from build123d import *

# Parameters (mm, degrees)
ESKIZ_KONTUR_W        = 3.2
ESKIZ_KONTUR_H        = 8.2
PLASTINA_DEPTH        = 3
OTVERSTIYA_DEPTH      = 49.541218109
OTVERSTIYA_DEPTH_BACK = 49.541218109
ESKIZ_OTVERSTIYA_R    = 0.75
ESKIZ_OTVERSTIYA_R_2  = 4.5
ESKIZ_OTVERSTIYA_R_3  = 3
ESKIZ_OTVERSTIYA_R_4  = 1.65


with BuildPart() as part:
    # Eskiz_kontur → Plastina (new body)
    with BuildSketch(Plane.XY):
        with BuildLine():
            Line((41.499998426, -24.999999723), (25.999998426, -24.999999723))
            Line((25.999998426, -24.999999723), (-4.976321574, -10.919529723))
            ThreePointArc((-4.976321574, -10.919529723), (-11.817691954, 2.083782335), (-0.94151, 11.96301))
            Line((-0.94151, 11.96301), (26, 14))
            Line((26, 14), (41.499998426, 14))
            Line((41.499998426, 14), (41.499998426, -24.999999723))
        make_face()
        with Locations((36.5, -16)):
            Rectangle(ESKIZ_KONTUR_W, ESKIZ_KONTUR_H, mode=Mode.SUBTRACT)
        with Locations((36.5, 6)):
            Rectangle(ESKIZ_KONTUR_W, ESKIZ_KONTUR_H, mode=Mode.SUBTRACT)
    extrude(amount=PLASTINA_DEPTH)

    # Eskiz_otverstiya → Otverstiya (cut, two sides: drawn at the far end of the back side and taken through both)
    with BuildSketch(Plane.XY.offset(-OTVERSTIYA_DEPTH_BACK)):
        with Locations((-7.77817, -7.77817)):
            Circle(ESKIZ_OTVERSTIYA_R)
        with Locations((-6.36396, -6.36396)):
            Circle(ESKIZ_OTVERSTIYA_R)
        with Locations((9.19239, -9.19239)):
            Circle(ESKIZ_OTVERSTIYA_R)
        with Locations((7.77817, -7.77817)):
            Circle(ESKIZ_OTVERSTIYA_R)
        with Locations((6.36396, -6.36396)):
            Circle(ESKIZ_OTVERSTIYA_R)
        with Locations((17, -8)):
            Circle(ESKIZ_OTVERSTIYA_R_2)
        with Locations((-4.94975, -4.94975)):
            Circle(ESKIZ_OTVERSTIYA_R)
        Circle(ESKIZ_OTVERSTIYA_R_3)
        with Locations((4.94975, -4.94975)):
            Circle(ESKIZ_OTVERSTIYA_R)
        with Locations((-4.94975, 4.94975)):
            Circle(ESKIZ_OTVERSTIYA_R)
        with Locations((-6.36396, 6.36396)):
            Circle(ESKIZ_OTVERSTIYA_R)
        with Locations((-7.77817, 7.77817)):
            Circle(ESKIZ_OTVERSTIYA_R)
        with Locations((4.94975, 4.94975)):
            Circle(ESKIZ_OTVERSTIYA_R)
        with Locations((6.36396, 6.36396)):
            Circle(ESKIZ_OTVERSTIYA_R)
        with Locations((7.77817, 7.77817)):
            Circle(ESKIZ_OTVERSTIYA_R)
        with Locations((9.19239, 9.19239)):
            Circle(ESKIZ_OTVERSTIYA_R)
        with Locations((36.5, -5)):
            Circle(ESKIZ_OTVERSTIYA_R_4)
    extrude(amount=OTVERSTIYA_DEPTH + OTVERSTIYA_DEPTH_BACK, mode=Mode.SUBTRACT)


solid = part.part
CAD build for the part. Positions are in the model's coordinates, mm. A direction names the side the tool comes from. Coordinates: 2 decimals unless noted, no trailing zeros. Order: outer loops, then holes, each group sorted by start corner. A loop starts at its lowest first (then second) coordinate and runs counter-clockwise, first axis right, second up. Notation, with made-up numbers: (-32.75, 43) -> (11.25, 43) arc R6 ccw to (11.25, 49) -> close; hole circle Ø11 at (-8.5, 25). An arc over 180 degrees is marked (long way). Answer in a Markdown table with one row per item.
1) Flat gauge pins, fed straight in: P1, Ø1.5, axis at y = 5, z = 1, coming from the -X side; P2, Ø1.5, axis at x = 1.5, z = 2.5, coming from the -Y side. Where does each tip first touch, or does it go through?
Check values:
| item | result |
|---|---|
| P1 | x = -11.22 |
| P2 | y = -14.2 |
2) Band-saw the part on C-C (z = 2.3). Give the number of separate pieces and of enclosed holes in the cut face, and give its area (3 significant figures).
Check values:
| item | result |
|---|---|
| separate pieces | 1 |
| enclosed holes | 19 |
| area | 1,490 mm2 |
3) Band-saw the part on A-A (x = 36.5). List the corners of the cut face in (y, z).
Check values:
| item | result |
|---|---|
| outline | (-25, 0) -> (-20.1, 0) -> (-20.1, 3) -> (-25, 3) -> close; (-11.9, 0) -> (-6.65, 0) -> (-6.65, 3) -> (-11.9, 3) -> close; (-3.35, 0) -> (1.9, 0) -> (1.9, 3) -> (-3.35, 3) -> close; (10.1, 0) -> (14, 0) -> (14, 3) -> (10.1, 3) -> close |
4) Which spindle directions (+Z, -Z, +X, -X, +Y, -Y) get a long thin tool onto all of the face, cutting with end or side? Do faces 1 (the face through (34.9, 6, 1)), 2 (the face through (-11.854, 1.865, 1.479)). Say none if no direction does.
Check values:
| item | result |
|---|---|
| face 1 | +Z, -Z |
| face 2 | +Z, -Z, -X |
5) Mould opens along Y. For faces 3 (the face through (21, -5, 3)), 4 (the face through (34, -25, 1)), 5 (the face through (-4.547, -4.317, 1.479)) say: pulls with the +Y half, pulls with the -Y half, needs draft (parallel to the pull), parting line crosses it, or undercut.
Check values:
| item | result |
|---|---|
| face 3 | needs draft |
| face 4 | pulls with the -Y half |
| face 5 | undercut |
6) Drill centre lines: line 1 (Y direction, x = 36.5, z = 1.4); line 2 (Y direction, x = 7.5, z = 2.5); line 3 (X direction, y = -4.5, z = 1). Where is each one in solid material? Low to high.
Check values:
| item | result |
|---|---|
| line 1 | -25 to -20.1, -11.9 to -6.65, -3.35 to 1.9, 10.1 to 14 |
| line 2 | -16.59 to -8.47, -7.08 to 7.08, 8.47 to 12.6 |
| line 3 | -11.12 to -5.55, -4.35 to 4.35, 5.55 to 14.17, 19.83 to 34.93, 38.07 to 41.5 |
7) Band-saw the part on D-D (x = 16.5). List the corners of the cut face in (y, z).
Check values:
| item | result |
|---|---|
| outline | (-20.68, 0) -> (-12.47, 0) -> (-12.47, 3) -> (-20.68, 3) -> close; (-3.53, 0) -> (13.28, 0) -> (13.28, 3) -> (-3.53, 3) -> close |
8) Band-saw the part on B-B (y = 0). List the corners of the cut face in (x, z), and give its area (4 significant figures).
Check values:
| item | result |
|---|---|
| outline | (-12, 0) -> (-3, 0) -> (-3, 3) -> (-12, 3) -> close; (3, 0) -> (41.5, 0) -> (41.5, 3) -> (3, 3) -> close |
| area | 142.5 mm2 |
